The model under review builds one solid part; all positions refer to its coordinate system, in mm. Round coordinates to 2 decimals unless told otherwise and drop trailing zeros. Order: outer loops, then holes, each group sorted by start corner. A loop starts at its lowest first (then second) coordinate and runs counter-clockwise, first axis right, second up.
1) Consider section D-D (x = -1.5). Give the boundary of the cut face in (y, z), then the cut area to 3 significant figures.
2) Consider section A-A (y = -10). Give the boundary of the cut face in (x, z).
3) Consider section C-C (z = 0.45). Give the number of separate pieces and of enclosed holes in the cut face, then the cut area to 3 significant figures.
4) Consider section B-B (x = -60). Give the boundary of the cut face in (y, z), then the cut area to 3 significant figures.
5) Clearance check with flat-ended pins moving along their axes: P1, Ø0.6, axis at y = -21.5, z = 2, coming from the -X side; P2, Ø1, axis at x = -56, z = 2, coming from the -Y side; P3, Ø0.9, axis at x = 5.5, z = 1, coming from the +Y side. State where each tip first meets the part, or that it passes through.
6) Mouldability with a two-part tool opening along X and no side actions: class faces 1 (the face through (1, 0, 3)), 2 (the face through (-68.331, -9.474, 1.479)), 3 (the face through (-68.331, 10.526, 1.479)) as pulls with the +X half, pulls with the -X half, needs draft (parallel to the pull), parting line crosses it, or undercut.
7) To check wall thickness, follow L1, parallel to Y at x = -60, z = 1.85; L2, parallel to Y at x = 65.5, z = 2.05. State the ranges of each line that lie inside material, in increasing order.
from build123d import *

# Parameters (mm, degrees)
SKETCH_R    = 1.75
PAD_DEPTH   = 3
FILLET_R    = 3
FILLET001_R = 1


with BuildPart() as part:
    # Sketch → Pad (new body)
    with BuildSketch(Plane.XY):
        Polygon((25.05, 23), (39.95, 23), (39.95, 20), (70.05, 20), (70.05, 23), (84.95, 23), (84.95, 20), (103.7, 20), (103.7, -20), (84.95, -20), (84.95, -23), (70.05, -23), (70.05, -20), (39.95, -20), (39.95, -23), (25.05, -23), (25.05, -20), (-25.05, -20), (-25.05, -23), (-39.95, -23), (-39.95, -20), (-70.05, -20), (-70.05, -23), (-84.95, -23), (-84.95, -20), (-103.7, -20), (-103.7, 20), (-84.95, 20), (-84.95, 23), (-70.05, 23), (-70.05, 20), (-39.95, 20), (-39.95, 23), (-25.05, 23), (-25.05, 20), (25.05, 20), align=None)
        with Locations((-70, 10)):
            Circle(SKETCH_R, mode=Mode.SUBTRACT)
        with Locations((-60, 10)):
            Circle(SKETCH_R, mode=Mode.SUBTRACT)
        with Locations((-70, -10)):
            Circle(SKETCH_R, mode=Mode.SUBTRACT)
        with Locations((-60, -10)):
            Circle(SKETCH_R, mode=Mode.SUBTRACT)
    extrude(amount=PAD_DEPTH)

    # Fillet
    fillet_edges = [part.edges().sort_by_distance(p)[0] for p in [
        (-103.7, 20, 1.5),
        (103.7, 20, 1.5),
        (103.7, -20, 1.5),
        (-103.7, -20, 1.5),
    ]]
    fillet(fillet_edges, radius=FILLET_R)

    # Fillet001
    fillet001_edges = [part.edges().sort_by_distance(p)[0] for p in [
        (-84.95, 23, 1.5),
        (-70.05, 23, 1.5),
        (-84.95, -23, 1.5),
        (-39.95, 23, 1.5),
        (-70.05, -23, 1.5),
        (-25.05, 23, 1.5),
        (-39.95, -23, 1.5),
        (25.05, 23, 1.5),
        (-25.05, -23, 1.5),
        (39.95, 23, 1.5),
        (25.05, -23, 1.5),
        (70.05, 23, 1.5),
        (39.95, -23, 1.5),
        (84.95, 23, 1.5),
        (70.05, -23, 1.5),
        (84.95, -23, 1.5),
    ]]
    fillet(fillet001_edges, radius=FILLET001_R)


solid = part.part
Answer below:
1. outline: (-20, 0) - (20, 0) - (20, 3) - (-20, 3) - close
1. area: 120 mm2
2. outline: (-103.7, 0) - (-71.75, 0) - (-71.75, 3) - (-103.7, 3) - close; (-68.25, 0) - (-61.75, 0) - (-61.75, 3) - (-68.25, 3) - close; (-58.25, 0) - (103.7, 0) - (103.7, 3) - (-58.25, 3) - close
3. separate pieces: 1
3. enclosed holes: 4
3. area: 8,600 mm2
4. outline: (-20, 0) - (-11.75, 0) - (-11.75, 3) - (-20, 3) - close; (-8.25, 0) - (8.25, 0) - (8.25, 3) - (-8.25, 3) - close; (11.75, 0) - (20, 0) - (20, 3) - (11.75, 3) - close
4. area: 99.0 mm2
5. P1: stops at x = -84.95
5. P2: stops at y = -20
5. P3: stops at y = 20
6. face 1: needs draft
6. face 2: undercut
6. face 3: undercut
7. L1: y = -20 to -11.75, -8.25 to 8.25, 11.75 to 20
7. L2: y = -20 to 20
